Print and shaded views of the part. All mm, measured from the part's lowest x, y and z. Round coordinates to 2 decimals unless told otherwise and drop trailing zeros. Loops run counter-clockwise (first coordinate to the right, second up) from the corner with the lowest first, then second, coordinate; pieces in that order, holes last. Notation, with made-up numbers: (22, 10) -> (72, 10) arc R15 ccw to (72, 35) -> close; hole circle Ø6 at (48, 42.25). An arc over 180 degrees is marked (long way). Use a Markdown table: item, result.
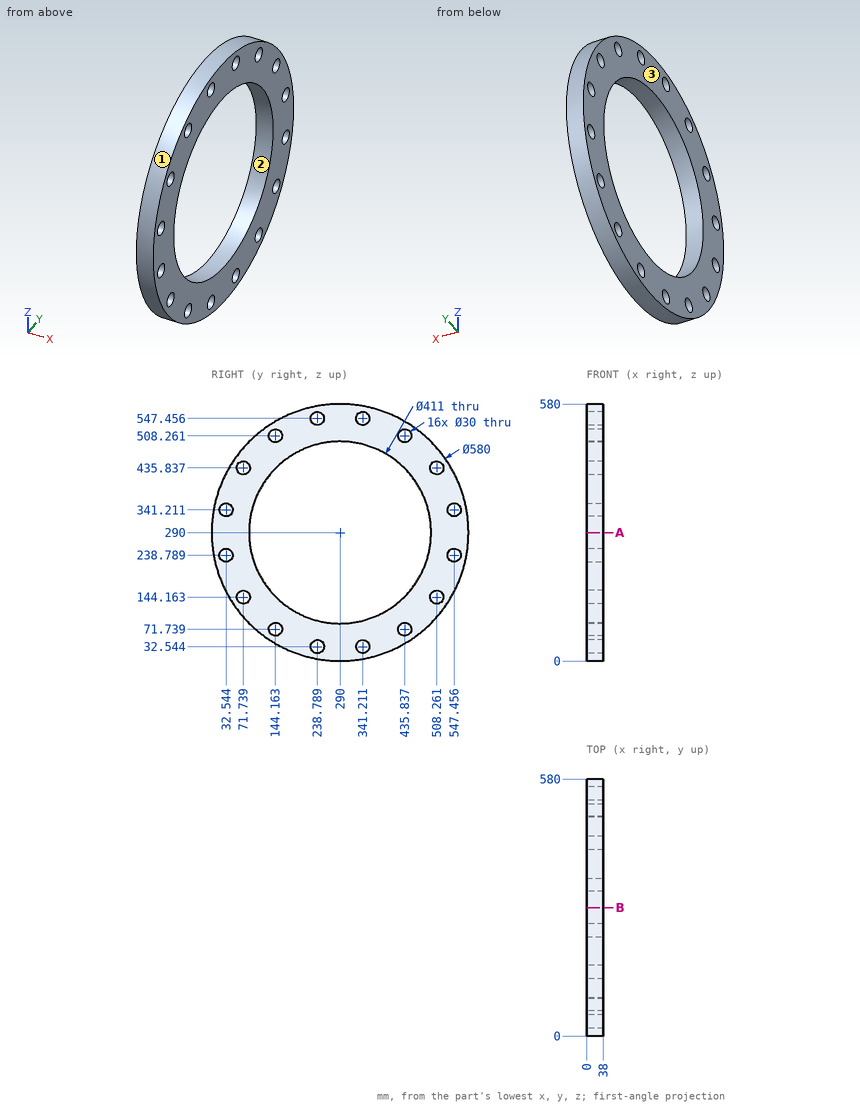
Q1. Flat gauge pins, fed straight in: pin 1 (18 mm diameter, centred on y = 435.84, z = 71.74, fed in from +X); pin 2 (10 mm diameter, centred on x = 23.5, z = 225, fed in from +Y) (1 decimal); pin 3 (8 mm diameter, centred on x = 27.5, y = 361, fed in from -Z); pin 4 (10 mm diameter, centred on x = 31, z = 398, fed in from +Y). Where does each tip first touch, or does it go through?
Results list:
| item | result |
|---|---|
| pin 1 | passes through |
| pin 2 | stops at y = 573.7 |
| pin 3 | stops at z = 7.85 |
| pin 4 | stops at y = 561.09 |
Q2. Band-saw the part on A-A, the plane z = 290. Give the cut face in (x, y).
Results list:
| item | result |
|---|---|
| outline | (0, 0) -> (38, 0) -> (38, 84.5) -> (0, 84.5) -> close; (0, 495.5) -> (38, 495.5) -> (38, 580) -> (0, 580) -> close |
Q3. Drill centre lines: L1, parallel to Y at x = 29.5, z = 355; L2, parallel to Z at x = 13, y = 290; L3, parallel to Z at x = 34.5, y = 455 (1 decimal). Where is each one in solid material? Low to high. Write a range as from..to.
Results list:
| item | result |
|---|---|
| L1 | y = 7.38..26.64, 38.45..95.05, 484.95..541.55, 553.36..572.62 |
| L2 | z = 0..84.5, 495.5..580 |
| L3 | z = 51.5..167.5, 412.5..528.5 |
Q4. Pull direction Y, two halves, no side cores. Call the marked faces 1, 2 and 3: released by +Y, released by -Y, zero draft, split by the parting line, or undercut.
Results list:
| item | result |
|---|---|
| face 1 | split by the parting line |
| face 2 | undercut |
| face 3 | zero draft |
